from build123d import *

# Parameters (mm, degrees)
F3_D = 5.588


with BuildPart() as f1:
    # F0 (on Front) → F1 (revolve)
    with BuildSketch(Plane.XZ):
        Polygon((-9.15198, 13.208), (-9.15198, 0), (4.56402, 0), (4.56402, 5.027528), (3.80202, 5.027528), (3.80202, 17.272), (0.75402, 17.272), (-0.486955, 13.208), (-1.650846, 13.208), (-2.506008, 17.272), (-3.522008, 17.272), (-5.248328, 13.208), (-6.465123, 13.208), (-6.86598, 17.272), (-8.00898, 17.272), (-8.00898, 13.208), align=None)
    revolve(axis=Axis((-2.29398, 0, 0), (1, 0, 0)))

    # F3 (through all)
    with Locations(Plane.YZ.offset(4.56402)):
        with Locations((0, 0)):
            Hole(F3_D / 2)


solid = f1.part
Geometry: final body of the model. Coordinates: model frame, mm. A direction names the side the tool comes from. Coordinates: 2 decimals unless noted, no trailing zeros. Order: outer loops, then holes, each group sorted by start corner. A loop starts at its lowest first (then second) coordinate and runs counter-clockwise, first axis right, second up.
1) Ray query, probe 1 along X at (y, z) = (11, 13); probe 2 along X at (y, z) = (1, -14) (3 decimals); probe 3 along X at (y, z) = (7.5, -9). Return the intervals inside material, ascending.
Result sheet:
probe 1: x = -8.01 to -6.84, -3.63 to -2.45, 0.68 to 3.8
probe 2: x = -8.009 to -6.547, -4.897 to -1.825, -0.234 to 3.802
probe 3: x = -9.15 to 3.8
2) Section C-C (x = 0). Return loops of the section in (y, z).
Result sheet:
outline: circle Ø29.61 at (0, 0); hole circle Ø5.59 at (0, 0)
3) Draft query along X for faces 1 (the flat face through (3.802, 4, -4)), 2 (the cylindrical face through (-5.87, 5.06, 12.2)), 3 (the cylindrical face through (-2.39, 2.217, -1.7)). Return one class per face: released by +X, released by -X, zero draft, split by the parting line, or undercut.
Result sheet:
face 1: released by +X
face 2: undercut
face 3: zero draft
4) Set-up query: faces 4 (the flat face through (-8.009, 13, -4)), 5 (the conical face through (-1.704, 13.142, -2.918)), 6 (the cylindrical face through (4.178, -4.985, -0.654)). Return all of +Z, -Z, +X, -X, +Y, -Y with unobstructed straight access to the full face (end or side cutting, diameter ignored); none if empty.
Result sheet:
face 4: -X
face 5: none
face 6: +X
5) First-contact query: P1, Ø1, axis at y = -12, z = 6.5, coming from the +X side; P2, Ø5, axis at x = -2.5, y = 4, coming from the +Z side; P3, Ø5, axis at x = 0.5, z = 8.5, coming from the +Y side. Flat tips, straight axial feed; report the tip coordinate or a pass-through.
Result sheet:
P1: stops at x = 3.8
P2: stops at z = 17.21
P3: stops at y = 16.19
